```python
from build123d import *

# Parameters (mm, degrees)
EXTRUDE_1_DEPTH     = 12
SKETCH_2_R          = 8
CUT_EXTRUDE_1_DEPTH = 8
SKETCH_3_R          = 2
CUT_EXTRUDE_2_DEPTH = 40


with BuildPart() as part:
    # 草图1 → 凸台-拉伸1 (new body)
    with BuildSketch(Plane(origin=(0, 0, 0), x_dir=(0, 0, -1), z_dir=(1, 0, 0))):
        with BuildLine():
            Line((-22.5, 15), (22.5, 15))
            ThreePointArc((22.5, 15), (26.035533906, 13.535533906), (27.5, 10))
            Line((27.5, 10), (27.5, -10))
            ThreePointArc((27.5, -10), (26.035533906, -13.535533906), (22.5, -15))
            Line((22.5, -15), (-22.5, -15))
            ThreePointArc((-22.5, -15), (-26.035533906, -13.535533906), (-27.5, -10))
            Line((-27.5, -10), (-27.5, 10))
            ThreePointArc((-27.5, 10), (-26.035533906, 13.535533906), (-22.5, 15))
        make_face()
    extrude(amount=EXTRUDE_1_DEPTH)

    # 草图2 → 切除-拉伸1 (cut)
    with BuildSketch(Plane.ZY):
        Circle(SKETCH_2_R)
    extrude(amount=-CUT_EXTRUDE_1_DEPTH, mode=Mode.SUBTRACT)

    # 草图3 → 切除-拉伸2 (cut)
    with BuildSketch(Plane.XZ.offset(15)):
        with Locations((4, 0)):
            Circle(SKETCH_3_R)
    extrude(amount=-CUT_EXTRUDE_2_DEPTH, mode=Mode.SUBTRACT)


solid = part.part
```
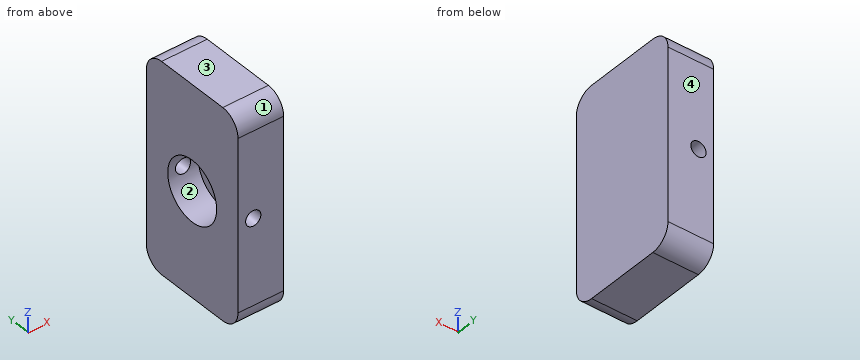
CAD build for the part. Positions are in the model's coordinates, mm. Face numbers are marked on the shaded views. Coordinates: 2 decimals unless noted, no trailing zeros. Order: outer loops, then holes, each group sorted by start corner. A loop starts at its lowest first (then second) coordinate and runs counter-clockwise, first axis right, second up.
(1) Saw through at D-D, the plane y = -9. Write the cut outline in (x, z).
Solution:
outline: (0, -27.5) - (12, -27.5) - (12, 27.5) - (0, 27.5) - close; hole circle Ø4 at (4, 0)
(2) Mould opens along Y. For the marked faces 1, 2, 3 and 4 say: released by +Y, released by -Y, zero draft, split by the parting line, or undercut.
Solution:
face 1: released by -Y
face 2: undercut
face 3: zero draft
face 4: released by +Y
(3) Drill centre lines: L1, parallel to Z at x = 4, y = 9.5; L2, parallel to X at y = 12, z = 0; L3, parallel to Y at x = 1.5, z = 2. Where is each one in solid material? Low to high.
Solution:
L1: z = -27.5 to -2, 2 to 27.5
L2: x = 0 to 2, 6 to 12
L3: y = -15 to -7.75, 7.75 to 15
(4) Pin check, flat tip, straight feed: pin 1 Ø3 at (y, z) = (-5, 14) entering from -X. Stop position of the tip, or through.
Solution:
pin 1: stops at x = 0
(5) Saw through at A-A, the plane x = 4. Write the cut outline in (y, z), and give its area (3 significant figures).
Solution:
outline: (-15, -22.5) arc R5 ccw to (-10, -27.5) - (10, -27.5) arc R5 ccw to (15, -22.5) - (15, -2) - (7.75, -2) arc R8 cw to (-7.75, -2) - (-15, -2) - close; (-15, 2) - (-7.75, 2) arc R8 cw to (7.75, 2) - (15, 2) - (15, 22.5) arc R5 ccw to (10, 27.5) - (-10, 27.5) arc R5 ccw to (-15, 22.5) - close
area: 1,370 mm2
(6) Saw through at B-B, the plane z = 0. Write the cut outline in (x, y), and give its area (3 significant figures).
Solution:
outline: (0, -15) - (2, -15) - (2, -8) - (0, -8) - close; (0, 8) - (2, 8) - (2, 15) - (0, 15) - close; (6, -15) - (12, -15) - (12, 15) - (6, 15) - (6, 8) - (8, 8) - (8, -8) - (6, -8) - close
area: 176 mm2
(7) Saw through at C-C, the plane y = 0. Write the cut outline in (x, z).
Solution:
outline: (0, -27.5) - (12, -27.5) - (12, 27.5) - (0, 27.5) - (0, 8) - (8, 8) - (8, -8) - (0, -8) - close
